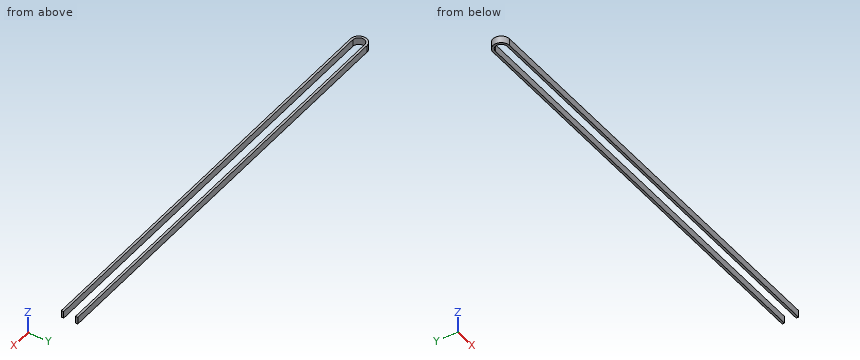
from build123d import *

# Parameters (mm, degrees)
SKETCH_1_W      = 370
SKETCH_1_H      = 6
EXTRUDE_1_DEPTH = 2
SKETCH_2_W      = 370
SKETCH_2_H      = 2
EXTRUDE_2_DEPTH = 6


with BuildPart() as part:
    # Эскиз1 → Бобышка-Вытянуть1 (new body)
    with BuildSketch(Plane(origin=(0, 0, 0), x_dir=(1, 0, 0), z_dir=(0, 1, 0))):
        with Locations((185, 3)):
            Rectangle(SKETCH_1_W, SKETCH_1_H)
    extrude(amount=EXTRUDE_1_DEPTH)

    # Эскиз2 → Бобышка-Вытянуть2 (add)
    with BuildSketch(Plane.XY):
        with BuildLine():
            ThreePointArc((0, 2), (-5, 7), (0, 12))
            Line((0, 12), (0, 14))
            ThreePointArc((0, 14), (-7, 7), (0, 0))
            Line((0, 0), (0, 2))
        make_face()
        with Locations((185, 13)):
            Rectangle(SKETCH_2_W, SKETCH_2_H)
    extrude(amount=-EXTRUDE_2_DEPTH)


solid = part.part
Source: CAD feature listing. Evaluate the final solid. Frame: model axes, mm. Give positions to 0.01 mm unless a question says otherwise; leave off trailing zeros. Loops run counter-clockwise (first coordinate to the right, second up) from the corner with the lowest first, then second, coordinate; pieces in that order, holes last. Notation, with made-up numbers: (60, 75.5) -> (88, 75.5) arc R35 ccw to (88, 111.5) -> close; hole circle Ø7 at (-13.75, 33.25). An arc over 180 degrees is marked (long way). Use a Markdown table: item, result. Add a question column.
1) Section query C-C, the plane y = 7. Return the cut outline in (x, z), then the cut area to 3 significant figures.
2) Line query: line 1 along Y through (x, z) = (167, -5.2); line 2 along X through (y, z) = (7.75, -1.2); line 3 along X through (y, z) = (13, -1.1). Output: solid intervals per line, ascending. Write a range as [from, to].
3) First-contact query: pin 1 (1 mm diameter, centred on y = 2.5, z = -3, fed in from -X); pin 2 (5 mm diameter, centred on x = 98.5, y = 8, fed in from -Z). Flat tips, straight axial feed; report the tip coordinate or a pass-through.
4) Section query A-A, the plane z = -3.45. Return the cut outline in (x, y).
5) Section query B-B, the plane x = 39. Return the cut outline in (y, z), then the cut area to 3 significant figures.
Numbers:
| question | item | result |
|---|---|---|
| 1 | outline | (-7, -6) -> (-5, -6) -> (-5, 0) -> (-7, 0) -> close |
| 1 | area | 12.0 mm2 |
| 2 | line 1 | y = [0, 2], [12, 14] |
| 2 | line 2 | x = [-6.96, -4.94] |
| 2 | line 3 | x = [-3.61, 370] |
| 3 | pin 1 | stops at x = -5.74 |
| 3 | pin 2 | passes through |
| 4 | outline | (0, 0) -> (370, 0) -> (370, 2) -> (0, 2) arc R5 cw to (0, 12) -> (370, 12) -> (370, 14) -> (0, 14) arc R7 ccw to start |
| 5 | outline | (0, -6) -> (2, -6) -> (2, 0) -> (0, 0) -> close; (12, -6) -> (14, -6) -> (14, 0) -> (12, 0) -> close |
| 5 | area | 24.0 mm2 |
